Check sheet for the modelled part. Datum: model origin and axes. Units: mm. A direction names the side the tool comes from. Give positions to 0.01 mm unless a question says otherwise; leave off trailing zeros. Write each loop counter-clockwise with the first axis right and the second up, starting at its lowest first coordinate (ties: lowest second). Pieces come first, ordered by that corner, then holes. Notation, with made-up numbers: (73.5, 62) -> (122.5, 62) arc R21 cw to (122.5, 80) -> close; hole circle Ø9 at (-17.5, -18). An arc over 180 degrees is marked (long way). Return JSON: item names as keys, results as strings.
from build123d import *

# Parameters (mm, degrees)
BOSS_EXTRUDE1_DEPTH = 2.5
SKETCH2_R           = 1.7
CUT_EXTRUDE1_DEPTH  = 1.5
FILLET1_R           = 1.5


with BuildPart() as part:
    # Sketch1 → Boss-Extrude1 (new body)
    with BuildSketch(Plane.XY):
        Polygon((-7.56419618, 12.7), (-7.56419618, 9.2), (5.44580382, 0), (5.44580382, 12.7), align=None)
    extrude(amount=BOSS_EXTRUDE1_DEPTH)

    # Sketch2 → Cut-Extrude1 (cut)
    with BuildSketch(Plane.XY.offset(2.5)):
        with Locations((-4.31419618, 9.2)):
            Circle(SKETCH2_R)
    extrude(amount=-CUT_EXTRUDE1_DEPTH, mode=Mode.SUBTRACT)

    # Mirror2: part across plane


with BuildPart() as part_1:
    add(part.part)
    add(part.part.mirror(Plane(origin=(5.44580382, 0, 2.5), x_dir=(0, 0, 1), z_dir=(-1, 0, 0))))

    # Fillet1
    fillet1_edges = [part_1.edges().sort_by_distance(p)[0] for p in [
        (18.45580382, 12.7, 1.25),
        (18.45580382, 9.2, 1.25),
        (5.44580382, 0, 1.25),
        (18.45580382, 10.95, 0),
        (11.95080382, 4.6, 0),
        (-1.05919618, 4.6, 0),
        (-7.56419618, 10.95, 0),
        (5.44580382, 12.7, 0),
        (-7.56419618, 12.7, 1.25),
    ]]
    fillet(fillet1_edges, radius=FILLET1_R)


solid = part_1.part
(1) Depth check by flat-ended pin: pin 1 Ø1.7 at (x, y) = (-4, 9.5) entering from +Z; pin 2 Ø5 at (x, y) = (15.5, 4.5) entering from +Z; pin 3 Ø1 at (x, z) = (7, 0.5) entering from +Y. Enter the tip coordinate at first touch or a pass-through.
Reply:
{"pin 1": "z = 1", "pin 2": "z = 2.5", "pin 3": "y = 12.61"}
(2) Cross-section at B-B on z = 0.45. Enter the section's corners in (x, y), then the cut area to 3 significant figures.
Reply:
{"outline": "(-7.14, 9.42) -> (4.83, 0.96) arc R1.07 ccw to (6.06, 0.96) -> (17.57, 9.1) arc R1.07 ccw to (18.03, 9.98) -> (18.03, 11.2) arc R1.07 ccw to (16.96, 12.27) -> (-6.06, 12.27) arc R1.07 ccw to (-7.14, 11.2) -> close", "area": "183 mm^2"}
(3) Set-up check for faces 4 (the cylindrical face through (16.904, 9.275, 1.76)), 5 (the cylindrical face through (18.293, 9.296, 2.007)): record each of +Z, -Z, +X, -X, +Y, -Y from which the full face is reachable in a straight line by a thin tool's end or side.
Reply:
{"face 4": "+Z", "face 5": "+Z, -Z, +X, -Y"}
(4) Release check for a two-part mould opening along X. For faces 1 (the flat face through (18.456, 11, 2)), 2 (the flat face through (-4, 9, 1)), 3 (the flat face through (-7.564, 10, 2)) record: pulls with the +X half, pulls with the -X half, needs draft (parallel to the pull), parting line crosses it, or undercut.
Reply:
{"face 1": "pulls with the +X half", "face 2": "undercut", "face 3": "pulls with the -X half"}
(5) Cross-section at A-A on z = 1.75. Enter the section's corners in (x, y).
Reply:
{"outline": "(-7.56, 9.2) -> (4.58, 0.61) arc R1.5 ccw to (6.31, 0.61) -> (17.82, 8.75) arc R1.5 ccw to (18.46, 9.98) -> (18.46, 11.2) arc R1.5 ccw to (16.96, 12.7) -> (-6.06, 12.7) arc R1.5 ccw to (-7.56, 11.2) -> close; hole circle Ø3.4 at (-4.31, 9.2); hole circle Ø3.4 at (15.21, 9.2)"}
(6) Thickness scan on L1, parallel to X at y = 10.75, z = 1.5; L2, parallel to X at y = 8.5, z = 2.35 (3 decimals); L3, parallel to Z at x = -5.25, y = 10. Record the ranges inside material, lowest first.
Reply:
{"L1": "-7.56 to -5.01, -3.62 to 14.51, 15.9 to 18.46", "L2": "-6.574 to -5.863, -2.765 to 13.657, 16.755 to 17.466", "L3": "0 to 1"}
